Autodesk Inventor part; units mm, degrees
ref_plane "YZ Plane" through (0, 0, 0) normal (1, 0, 0) x (0, 1, 0)
ref_plane "XZ Plane" through (0, 0, 0) normal (0, 1, 0) x (-1, 0, 0)
ref_plane "XY Plane" through (0, 0, 0) normal (0, 0, 1) x (1, 0, 0)
sketch "Sketch3" plane through (0, 0, 0) normal (1, 0, 0) x (0, 1, 0)
  line L0 (6, 19.5) -> (0, 19.5)
  line L1 (0, 19.5) -> (0, -19.5)
  line L2 (0, -19.5) -> (6, -19.5)
  line L3 (6, -19.5) -> (6, 19.5)
  point P0 (0, 0)
  dimension "d11" = 39
  dimension "d12" = 0
  dimension "d13" = 6
  dimension "d15" = 19.5
revolve "Revolution2" add sketch "Sketch3" angle 360 about axis through (0, 0, 19.5) along (0, 0, -1)
sketch "Sketch6" plane through (0, 0, -19.5) normal (0, 0, -1) x (-1, 0, 0)
  circle A0 centre (0, 0) radius 2.5
  dimension "d39" = 5
hole "Hole3" at (0, 0, -19.5) direction (0, 0, 1) diameter 5 depth 14 tip angle 118
sketch "Sketch7" plane through (0, 0, 0) normal (0, 1, 0) x (-1, 0, 0)
  circle A0 centre (0, -14.5) radius 2
  line L0 (-6, -19.5) -> (6, -19.5)
  point P0 (0, 0)
  dimension "d47" = 4
  dimension "d49" = 5
hole "Hole4" at (0, 0, -14.5) direction (0, -1, 0) diameter 3.242 end through all
thread "Thread2"
chamfer "Chamfer3" distance 1.5 angle 45 1 edges at (0, -6, 19.5)
equation "\"d40\" = d39"
properties part number "Spindle Iso M12 Setscrew" material "Aluminum 6061"
Could you check a few things on this model? Use its own coordinates, in mm. A direction names the side the tool comes from. Give positions to 0.01 mm unless a question says otherwise; leave off trailing zeros. Order: outer loops, then holes, each group sorted by start corner. A loop starts at its lowest first (then second) coordinate and runs counter-clockwise, first axis right, second up.
Q1. If I drill on line 1 along Z through (x, y) = (0, -3.9); line 2 along Y through (x, z) = (0, -12.5), over which ranges is the centre line in solid material (lowest first)?
Q2. Suppose I cut it at C-C, the plane z = -14.5. Write out the boundary of the cut face in (x, y).
Q3. We'd pull the mould along Y, two halves only. Please class faces 4 (the cylindrical face through (-1.802, 5.723, -0.488)), 5 (the conical face through (0, 0, -4)), 6 (the flat face through (0, 3, -19.5)): +Y half, -Y half, draft (parallel to the pull), parting line (faces both ways), or undercut.
Q4. I'm going to push flat-ended pins straight in: P1, Ø1, axis at y = -2.5, z = -12, coming from the -X side; P2, Ø1, axis at x = -4.5, z = -11.5, coming from the -Y side; P3, Ø2, axis at x = 3, z = 6, coming from the -Y side; P4, Ø6, axis at x = -1.5, z = 2.5, coming from the -Y side. Where does each tip first touch, or does it pass through?
Q5. For faces 1 (the cylindrical face through (0.621, -3.981, -13.003)), 2 (the conical face through (0, -5, 19)), 3 (the cylindrical face through (-0.751, 2.385, -12.402)), which set-ups out of +Z, -Z, +X, -X, +Y, -Y let a thin tool reach every point of the face, with its end or its side?
Q6. Suppose I cut it at A-A, the plane z = -9. Write out the boundary of the cut face in (x, y), and give its area (3 significant figures).
Q7. Suppose I cut it at B-B, the plane z = 16. Write out the boundary of the cut face in (x, y).
Solution:
1. line 1: z = -19.5 to -16.12, -12.88 to 19.5
1. line 2: y = -6 to -2.5, 2.5 to 6
2. outline: (-1.62, -5.78) - (-1.62, -1.9) arc R2.5 cw (long way) to (1.62, -1.9) - (1.62, -5.78) arc R6 ccw (long way) to start
3. face 4: parting line
3. face 5: undercut
3. face 6: draft
4. P1: stops at x = -5.66
4. P2: stops at y = -4.47
4. P3: stops at y = -5.66
4. P4: stops at y = -6
5. face 1: -Y
5. face 2: +Z
5. face 3: -Z
6. outline: circle Ø12 at (0, 0); hole circle Ø5 at (0, 0)
6. area: 93.5 mm2
7. outline: circle Ø12 at (0, 0)
